Input: dimensioned drawing with shaded views. Units: mm. Origin: part minimum x, y, z. A direction names the side the tool comes from. Round coordinates to 2 decimals unless told otherwise and drop trailing zeros. Order: outer loops, then holes, each group sorted by start corner. A loop starts at its lowest first (then second) coordinate and runs counter-clockwise, first axis right, second up. Notation, with made-up numbers: (71.25, 55) - (116.25, 55) arc R21 ccw to (116.25, 73) - close; hole circle Ø4 at (40, 80.5). An arc over 180 degrees is marked (long way). Put each result on its own line as item: value. Start each with the question number.
(1) Section B-B (x = 19.5). Output: boundary loops of the cut face in (y, z).
(2) Section A-A (z = 3.5). Output: boundary loops of the cut face in (x, y), and give its area (3 significant figures).
(3) Section C-C (y = 29). Output: boundary loops of the cut face in (x, z), and give its area (3 significant figures).
(4) Pin query (flat end, axial travel): P1, Ø9, axis at x = 51.5, z = 31, coming from the -Y side; P2, Ø2, axis at x = 35, z = 32, coming from the -Y side; P3, Ø7, axis at x = 42.5, y = 36.5, coming from the +Z side; P4, Ø5, axis at x = 48, y = 7, coming from the +Z side. Return the tip coordinate at first contact, or that it passes through.
(5) Pull-direction query (X, two-part tool) for the marked faces 1, 2, 3 and 4; classes: released by +X, released by -X, zero draft, split by the parting line, or undercut.
(6) Material intervals for L1, parallel to X at y = 32, z = 25.5; L2, parallel to X at y = 35.5, z = 31.5; L3, parallel to Y at x = 62.5, z = 4.5, sorted ascending. Write a range as [from, to].
(7) Access query for the marked faces 5, 6 and 7. Directions: +Z, -Z, +X, -X, +Y, -Y. A direction counts if a zero-diameter tool reaches every point of the face in a straight line with its end or side. Return the directions, or none.
(8) Section D-D (x = 52.5). Output: boundary loops of the cut face in (y, z), and give its area (3 significant figures).
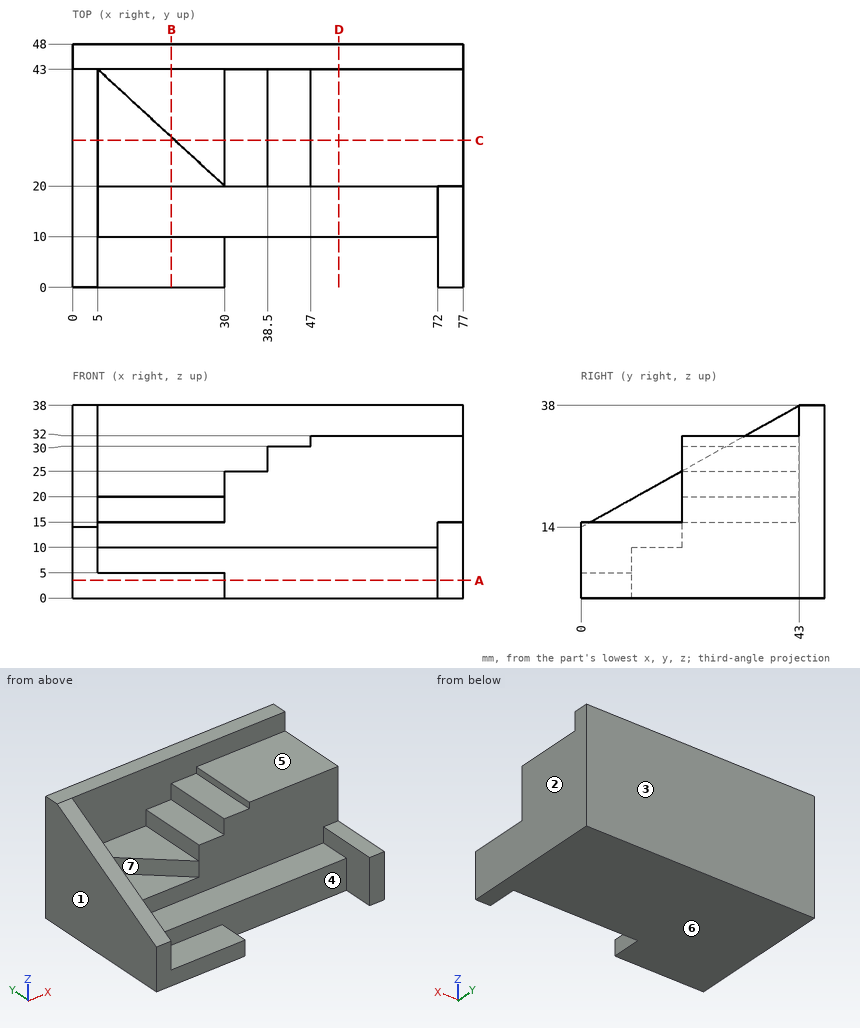
Checks:
1. outline: (0, 0) - (48, 0) - (48, 38) - (43, 38) - (43, 20) - (29.66, 20) - (29.66, 15) - (20, 15) - (20, 10) - (10, 10) - (10, 5) - (0, 5) - close
2. outline: (0, 0) - (30, 0) - (30, 10) - (72, 10) - (72, 0) - (77, 0) - (77, 48) - (0, 48) - close
2. area: 3,280 mm²
3. outline: (0, 0) - (77, 0) - (77, 32) - (47, 32) - (47, 30) - (38.5, 30) - (38.5, 25) - (30, 25) - (30, 20) - (20.22, 20) - (20.22, 15) - (5, 15) - (5, 30.19) - (0, 30.19) - close
3. area: 2,000 mm²
4. P1: stops at y = 20
4. P2: stops at y = 43
4. P3: stops at z = 30
4. P4: passes through
5. face 1: released by -X
5. face 2: released by +X
5. face 3: zero draft
5. face 4: undercut
6. L1: x = [0, 5], [38.5, 77]
6. L2: x = [0, 5], [47, 77]
6. L3: y = [10, 48]
7. face 5: +Z, +X, -Y
7. face 6: -Z, +X, -X, +Y, -Y
7. face 7: +Z, -Y
8. outline: (10, 0) - (48, 0) - (48, 38) - (43, 38) - (43, 32) - (20, 32) - (20, 10) - (10, 10) - close
8. area: 1,030 mm²
